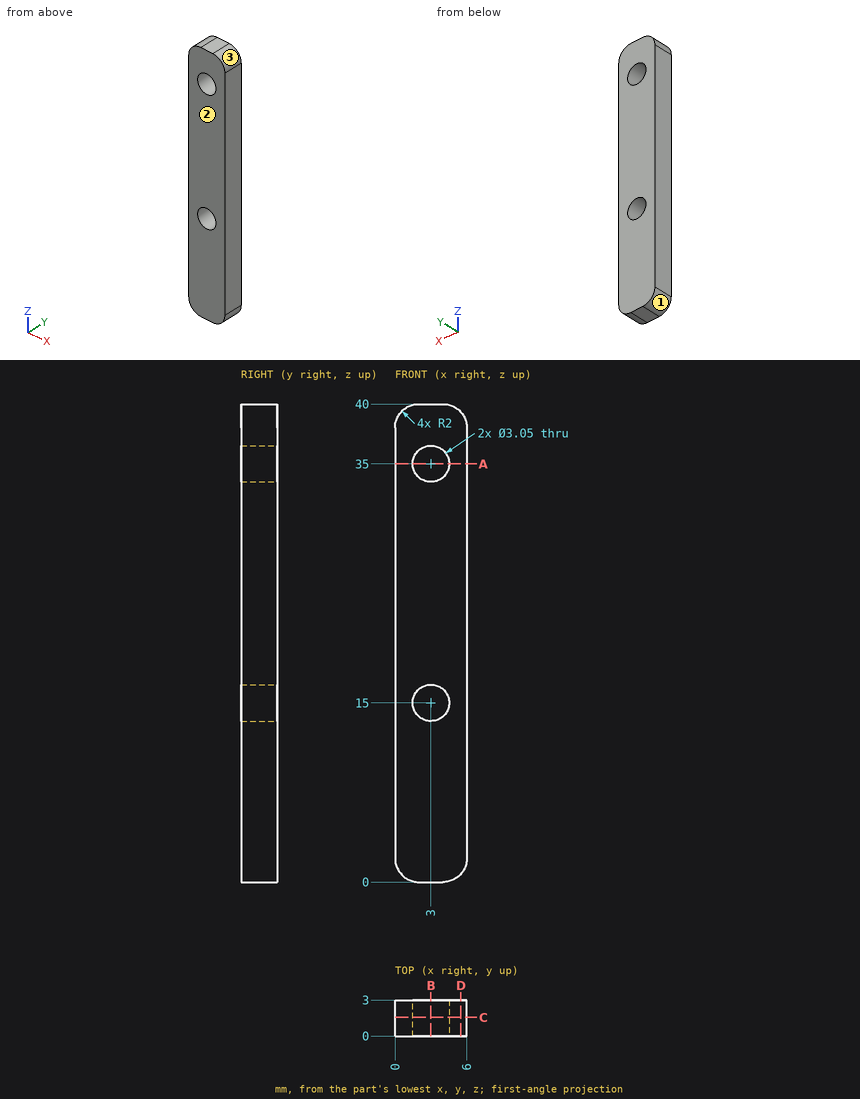
Geometry: see drawing. Coordinates: mm, zero at the bounding-box minimum. Coordinates: 2 decimals unless noted, no trailing zeros. Order: outer loops, then holes, each group sorted by start corner. A loop starts at its lowest first (then second) coordinate and runs counter-clockwise, first axis right, second up. Notation, with made-up numbers: M 44,-14.75 L 92,-14.75 A13 ccw 92,9.25 Z; hole C 64,29 d2. An arc over 180 degrees is marked long. Answer in a Markdown table with one row per item. Add a question column.
Q1. Section query B-B on x = 3. Return the cut outline in (y, z) (3 decimals).
Q2. Contact query for a flat-ended pin moving along its axis: P1, Ø2, axis at x = 3.5, z = 6, coming from the -Y side. Output: stop coordinate, or through.
Q3. Mould query, pull axis X, two halves, no side actions, for the marked faces 1, 2 and 3. Classes: released by +X, released by -X, zero draft, split by the parting line, or undercut.
Q4. Section query A-A on z = 35. Return the cut outline in (x, y) (3 decimals), and give its area (3 significant figures).
Q5. Section query D-D on x = 5.5. Return the cut outline in (y, z), and give its area (3 significant figures).
Q6. Section query C-C on y = 1.55. Return the cut outline in (x, z) (3 decimals).
Q7. Line query: L1, parallel to Z at x = 3, y = 1.05 (3 decimals); L2, parallel to X at y = 2.05, z = 35 (3 decimals); L3, parallel to Z at x = 1.75, y = 2.85. Output: solid intervals per line, ascending.
Completed:
| question | item | result |
|---|---|---|
| 1 | outline | M 0,0 L 3,0 L 3,13.475 L 0,13.475 Z; M 0,16.525 L 3,16.525 L 3,33.475 L 0,33.475 Z; M 0,36.525 L 3,36.525 L 3,40 L 0,40 Z |
| 2 | P1 | stops at y = 0 |
| 3 | face 1 | released by -X |
| 3 | face 2 | zero draft |
| 3 | face 3 | released by +X |
| 4 | outline | M 0,0 L 1.475,0 L 1.475,3 L 0,3 Z; M 4.525,0 L 6,0 L 6,3 L 4.525,3 Z |
| 4 | area | 8.85 mm2 |
| 5 | outline | M 0,0.68 L 3,0.68 L 3,39.32 L 0,39.32 Z |
| 5 | area | 116 mm2 |
| 6 | outline | M 0,2 A2 ccw 2,0 L 4,0 A2 ccw 6,2 L 6,38 A2 ccw 4,40 L 2,40 A2 ccw 0,38 Z; hole C 3,15 d3.05; hole C 3,35 d3.05 |
| 7 | L1 | z = 0 to 13.475, 16.525 to 33.475, 36.525 to 40 |
| 7 | L2 | x = 0 to 1.475, 4.525 to 6 |
| 7 | L3 | z = 0.02 to 14.13, 15.87 to 34.13, 35.87 to 39.98 |
